Work out the finished part from the listing and answer in its coordinate system (mm). A direction names the side the tool comes from. Coordinates: 2 decimals unless noted, no trailing zeros. Loops run counter-clockwise (first coordinate to the right, second up) from the corner with the lowest first, then second, coordinate; pieces in that order, holes last.
```python
from build123d import *

# Parameters (mm, degrees)
AUFSATZ_LINEAR_AUSTRAGEN1_DEPTH = 10
FASE1_SIZE                      = 5
SKIZZE2_R                       = 1.6
SCHNITT_LINEAR_AUSTRAGEN1_DEPTH = 10
SKIZZE3_R                       = 2.5
SKIZZE3_R_2                     = 1.6
AUFSATZ_LINEAR_AUSTRAGEN2_DEPTH = 10
SKIZZE5_R                       = 2.5
SKIZZE5_R_2                     = 1.6
AUFSATZ_LINEAR_AUSTRAGEN3_DEPTH = 10
SKIZZE4_R                       = 1.6
SCHNITT_LINEAR_AUSTRAGEN3_DEPTH = 10


with BuildPart() as part:
    # Skizze1 → Aufsatz-Linear austragen1 (new body)
    with BuildSketch(Plane.XY):
        Polygon((0, 30), (10, 30), (10, 10), (30, 10), (30, 0), (0, 0), align=None)
    extrude(amount=AUFSATZ_LINEAR_AUSTRAGEN1_DEPTH)

    # Fase1
    fase1_edges = [part.edges().sort_by_distance(p)[0] for p in [
        (10, 30, 5),
        (30, 10, 5),
    ]]
    chamfer(fase1_edges, length=FASE1_SIZE)

    # Skizze2 → Schnitt-Linear austragen1 (cut)
    with BuildSketch(Plane.ZY):
        with Locations((5, 15)):
            Circle(SKIZZE2_R)
        with Locations((5, 25)):
            Circle(SKIZZE2_R)
    extrude(amount=-SCHNITT_LINEAR_AUSTRAGEN1_DEPTH, mode=Mode.SUBTRACT)

    # Skizze3 → Aufsatz-Linear austragen2 (add)
    with BuildSketch(Plane.ZY):
        with Locations((5, 25)):
            Circle(SKIZZE3_R)
        with Locations((5, 25)):
            Circle(SKIZZE3_R_2, mode=Mode.SUBTRACT)
    extrude(amount=-AUFSATZ_LINEAR_AUSTRAGEN2_DEPTH)

    # Skizze5 → Aufsatz-Linear austragen3 (add)
    with BuildSketch(Plane.XZ):
        with Locations((25, 5)):
            Circle(SKIZZE5_R)
        with Locations((25, 5)):
            Circle(SKIZZE5_R_2, mode=Mode.SUBTRACT)
    extrude(amount=-AUFSATZ_LINEAR_AUSTRAGEN3_DEPTH)

    # Skizze4 → Schnitt-Linear austragen3 (cut)
    with BuildSketch(Plane.XZ):
        with Locations((15, 5)):
            Circle(SKIZZE4_R)
        with Locations((25, 5)):
            Circle(SKIZZE4_R)
    extrude(amount=-SCHNITT_LINEAR_AUSTRAGEN3_DEPTH, mode=Mode.SUBTRACT)


solid = part.part
```
1. Each of these flat-tipped pins is pushed along its axis until it touches: P1, Ø3, axis at x = 13, z = 8.5, coming from the -Y side; P2, Ø3, axis at x = 16.5, z = 7.5, coming from the +Y side; P3, Ø2, axis at y = 15, z = 3.5, coming from the +X side; P4, Ø2.5, axis at y = 25, z = 5, coming from the +X side. Where does it stop, or does it pass through?
2. Straight lines are drawn through the part: probe 1 along Y at (x, z) = (4, 5); probe 2 along Z at (x, y) = (25, 5.25); probe 3 along X at (y, z) = (21.25, 5.25). For each, find the intervals that lie inside material, in ascending order.
3. A cutting plane is placed at C-C, the plane z = 8.5. Give the vertices of the cut face in (x, y), then the cut area to 3 significant figures.
4. A cutting plane is placed at A-A, the plane y = 15. Give the vertices of the cut face in (x, z), then the cut area to 3 significant figures.
5. For faces 1 (the cylindrical face through (26.485, 4.93, 5.595)), 2 (the flat face through (10, 19, 5)), 3 (the cylindrical face through (27.5, 9, 4.9)), determine the directions among +Z, -Z, +X, -X, +Y, -Y from which every point of the face is accessible in a straight line to the end or side of a thin tool.
6. A cutting plane is placed at D-D, the plane y = 5.5. Give the vertices of the cut face in (x, z).
7. Determine the mould class of faces 4 (the cylindrical face through (13.4, 4.93, 5.07)), 5 (the flat face through (28, 7, 5)), 6 (the cylindrical face through (4.93, 24.03, 3.73)), 7 (the flat face through (9, 12, 10)) for opening direction Z: released by +Z, released by -Z, zero draft, split by the parting line, or undercut.
Answers below:
1. P1: stops at y = 0
1. P2: stops at y = 10
1. P3: stops at x = 10
1. P4: passes through
2. probe 1: y = 0 to 13.4, 16.6 to 23.4, 26.6 to 30
2. probe 2: z = 0 to 3.4, 6.6 to 10
2. probe 3: x = 0 to 10
3. outline: (0, 0) - (30, 0) - (30, 5) - (25, 10) - (10, 10) - (10, 25) - (5, 30) - (0, 30) - close
3. area: 475 mm2
4. outline: (0, 0) - (10, 0) - (10, 3.4) - (0, 3.4) - close; (0, 6.6) - (10, 6.6) - (10, 10) - (0, 10) - close
4. area: 68.0 mm2
5. face 1: +Y, -Y
5. face 2: +Z, -Z, +X, +Y
5. face 3: +X, +Y
6. outline: (0, 0) - (29.5, 0) - (29.5, 10) - (0, 10) - close; hole circle Ø3.2 at (15, 5); hole circle Ø3.2 at (25, 5)
7. face 4: undercut
7. face 5: zero draft
7. face 6: undercut
7. face 7: released by +Z
